Geometry check sheet. Reference: the model listing, model coordinates, mm. Face numbers are marked on the shaded views. A direction names the side the tool comes from. Give positions to 0.01 mm unless a question says otherwise; leave off trailing zeros. Loops run counter-clockwise (first coordinate to the right, second up) from the corner with the lowest first, then second, coordinate; pieces in that order, holes last. Notation, with made-up numbers: (-39.75, 82.25) -> (-1.75, 82.25) arc R5 cw to (-1.75, 86.25) -> close; hole circle Ø8 at (66.25, 42.25). An arc over 180 degrees is marked (long way). One line per item, written item: value. Start each with the question number.
(1) Sectioned sample at B-B, the plane x = 0. Record the cut outline in (y, z).
(2) Sectioned sample at D-D, the plane y = 9. Record the cut outline in (x, z).
(3) Sectioned sample at C-C, the plane x = 19.05. Record the cut outline in (y, z), then the cut area to 3 significant figures.
(4) Sectioned sample at A-A, the plane y = 0. Record the cut outline in (x, z).
(5) Tool access check on the marked faces 1 and 2. Record the directions out of +Z, -Z, +X, -X, +Y, -Y that give a thin tool (end or side, any length) a straight path to the whole face; none if there is none.
(6) Gauge pin test, flat ends, axial feed: pin 1 Ø5 at (x, y) = (-24.5, 27.5) entering from -Z; pin 2 Ø5 at (y, z) = (4.5, 2.5) entering from +X (3 decimals); pin 3 Ø5 at (y, z) = (-32, 8) entering from -X; pin 4 Ø8 at (x, y) = (1.5, -9) entering from +Z. Record the tip position at first contact, or that the pin passes through.
(7) Draft check along X on the marked faces 3, 4 and 5. Enter one of: pulls with the +X half, pulls with the -X half, needs draft (parallel to the pull), parting line crosses it, or undercut.
(8) Scan lines: line 1 along Y through (x, z) = (19.05, 3.75); line 2 along Y through (x, z) = (20, 6.5); line 3 along Y through (x, z) = (0, 6). Record each from-to range of solid material in increasing order. Write a range as from..to.
from build123d import *

# Parameters (mm, degrees)
SKETCH1_R           = 44.45
BOSS_EXTRUDE1_DEPTH = 9.7
SKETCH2_R           = 16
CUT_EXTRUDE1_DEPTH  = 6.7
SKETCH3_R           = 11
CUT_EXTRUDE2_DEPTH  = 9
SKETCH5_R           = 2
CUT_EXTRUDE4_DEPTH  = 10.7


with BuildPart() as part:
    # Sketch1 → Boss-Extrude1 (new body)
    with BuildSketch(Plane.XY):
        Circle(SKETCH1_R)
    extrude(amount=BOSS_EXTRUDE1_DEPTH)

    # Sketch2 → Cut-Extrude1 (cut)
    with BuildSketch(Plane.XY.offset(9.7)):
        Circle(SKETCH2_R)
    extrude(amount=-CUT_EXTRUDE1_DEPTH, mode=Mode.SUBTRACT)

    # Sketch3 → Cut-Extrude2 (cut)
    with BuildSketch(Plane.XY.offset(3)):
        Circle(SKETCH3_R)
    extrude(amount=-CUT_EXTRUDE2_DEPTH, mode=Mode.SUBTRACT)

    # Sketch5 → Cut-Extrude4 (cut, through all)
    with BuildSketch(Plane(origin=(0, 0, 0), x_dir=(-1, 0, 0), z_dir=(0, 0, -1))):
        with Locations((38.1, 0)):
            Circle(SKETCH5_R)
        with Locations((-19.05, -32.995567884)):
            Circle(SKETCH5_R)
        with Locations((-19.05, 32.995567884)):
            Circle(SKETCH5_R)
    extrude(amount=-CUT_EXTRUDE4_DEPTH, mode=Mode.SUBTRACT)


solid = part.part
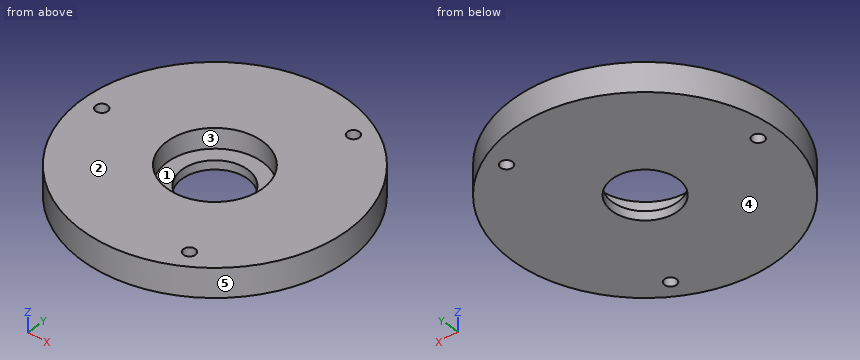
Calculated:
1. outline: (-44.45, 0) -> (-11, 0) -> (-11, 3) -> (-16, 3) -> (-16, 9.7) -> (-44.45, 9.7) -> close; (11, 0) -> (44.45, 0) -> (44.45, 9.7) -> (16, 9.7) -> (16, 3) -> (11, 3) -> close
2. outline: (-43.53, 0) -> (-6.32, 0) -> (-6.32, 3) -> (-13.23, 3) -> (-13.23, 9.7) -> (-43.53, 9.7) -> close; (6.32, 0) -> (43.53, 0) -> (43.53, 9.7) -> (13.23, 9.7) -> (13.23, 3) -> (6.32, 3) -> close
3. outline: (-40.16, 0) -> (-35, 0) -> (-35, 9.7) -> (-40.16, 9.7) -> close; (-31, 0) -> (31, 0) -> (31, 9.7) -> (-31, 9.7) -> close; (35, 0) -> (40.16, 0) -> (40.16, 9.7) -> (35, 9.7) -> close
3. area: 702 mm2
4. outline: (-44.45, 0) -> (-40.1, 0) -> (-40.1, 9.7) -> (-44.45, 9.7) -> close; (-36.1, 0) -> (-11, 0) -> (-11, 3) -> (-16, 3) -> (-16, 9.7) -> (-36.1, 9.7) -> close; (11, 0) -> (44.45, 0) -> (44.45, 9.7) -> (16, 9.7) -> (16, 3) -> (11, 3) -> close
5. face 1: +Z
5. face 2: +Z, +X, -X, +Y, -Y
6. pin 1: stops at z = 0
6. pin 2: stops at x = 44.405
6. pin 3: stops at x = -33.25
6. pin 4: stops at z = 3
7. face 3: undercut
7. face 4: needs draft
7. face 5: parting line crosses it
8. line 1: y = -40.16..-35, -31..31, 35..40.16
8. line 2: y = -39.7..-34.76, -31.24..31.24, 34.76..39.7
8. line 3: y = -44.45..-16, 16..44.45
